Input: part model. Units: mm. Frame: model coordinates. Face numbers are marked on the shaded views. A direction names the side the tool comes from. Coordinates: 2 decimals unless noted, no trailing zeros. Loops run counter-clockwise (first coordinate to the right, second up) from the corner with the lowest first, then second, coordinate; pieces in that order, holes last.
Item 1: Pull-direction query (Z, two-part tool) for the marked faces 6, 7, 8 and 9; classes: released by +Z, released by -Z, zero draft, split by the parting line, or undercut.
Item 2: Ray query, line 1 along Z through (x, y) = (12.5, -0.25); line 2 along Z through (x, y) = (7, -4); line 3 along Y through (x, z) = (16, -21). Return the intervals inside material, ascending.
Item 3: Section D-D on x = 15. Return loops of the section in (y, z).
Item 4: Section A-A on z = -12.5. Return loops of the section in (x, y).
Item 5: Contact query for flat-ended pins moving along their axis: P1, Ø2, axis at x = 13.5, y = -2.5, coming from the +Z side; P2, Ø10, axis at x = 14, z = -12, coming from the -Y side; P3, Ø10, axis at x = 21, z = -16, coming from the -Y side; P4, Ø3, axis at x = 23.5, y = -2.5, coming from the -Z side. Output: stop coordinate, or through.
Item 6: Section C-C on x = 25. Return loops of the section in (y, z), and give its area (3 significant figures).
Item 7: Section B-B on y = -5.75. Return loops of the section in (x, z).
Item 8: Reachability of the marked faces 1, 2, 3, 4 and 5 from +Z, -Z, +X, -X, +Y, -Y: full face, straight path, thin tool, end or side. Return the list, or none.
```python
from build123d import *

# Parameters (mm, degrees)
BOSS_EXTRUDE1_DEPTH = 2
BOSS_EXTRUDE2_DEPTH = 2
SKETCH3_R           = 1
BOSS_EXTRUDE3_DEPTH = 2.5
SKETCH5_R           = 1
BOSS_EXTRUDE5_DEPTH = 2.5
SKETCH6_R           = 1
CUT_EXTRUDE1_DEPTH  = 2.5
BOSS_EXTRUDE6_START = -2.5
SKETCH8_R           = 1
BOSS_EXTRUDE6_DEPTH = 2.5
CUT_EXTRUDE2_DEPTH  = 2.5
SKETCH10_R          = 9.941576331
SKETCH10_R_2        = 9.5
BOSS_EXTRUDE9_DEPTH = 2.5


with BuildPart() as part:
    # Sketch1 → Boss-Extrude1 (new body)
    with BuildSketch(Plane(origin=(0, 0, 0), x_dir=(1, 0, 0), z_dir=(0, 1, 0))):
        Polygon((0, 2.5), (0, 0), (26, 0), (26, 25), (0, 25), (0, 22.5), (5, 22.5), (5, 2.5), align=None)
    extrude(amount=BOSS_EXTRUDE1_DEPTH)

    # Sketch2 → Boss-Extrude2 (add)
    with BuildSketch(Plane(origin=(0, 2, 0), x_dir=(1, 0, 0), z_dir=(0, 1, 0))):
        Polygon((26, 25), (40.579221248, 15.4966373), (40.579221248, 9.198619924), (26, 0), align=None)
    extrude(amount=-BOSS_EXTRUDE2_DEPTH)

    # Sketch3 → Boss-Extrude3 (add)
    with BuildSketch(Plane.XY):
        Polygon((15.962952465, 0), (0, 0), (0, -7.986136178), (3.187790207, -7.986136178), align=None)
        with Locations((1.984518411, -4.657937593)):
            Circle(SKETCH3_R, mode=Mode.SUBTRACT)
    extrude(amount=-BOSS_EXTRUDE3_DEPTH)

    # Sketch5 → Boss-Extrude5 (add)
    with BuildSketch(Plane.XY):
        with Locations((1.984518411, -4.657937593)):
            Circle(SKETCH5_R)
    extrude(amount=-BOSS_EXTRUDE5_DEPTH)

    # Sketch6 → Cut-Extrude1 (cut)
    with BuildSketch(Plane.XY):
        with Locations((1.984518411, -3.146677254)):
            Circle(SKETCH6_R)
    extrude(amount=-CUT_EXTRUDE1_DEPTH, mode=Mode.SUBTRACT)

    # Sketch8 → Boss-Extrude6 (add)
    with BuildSketch(Plane(origin=(0, 0, -25), x_dir=(-1, 0, 0), z_dir=(0, 0, -1)).offset(BOSS_EXTRUDE6_START)):
        Polygon((0, 0), (0, -7.986136178), (-3.187790207, -7.986136178), (-15.962952465, 0), align=None)
        with Locations(Location((-1.984518411, -3.146677254, 0), (0, 0, 180))):
            Circle(SKETCH8_R, mode=Mode.SUBTRACT)
    extrude(amount=BOSS_EXTRUDE6_DEPTH)

    # Sketch9 → Cut-Extrude2 (cut)
    with BuildSketch(Plane(origin=(0, 2, 0), x_dir=(1, 0, 0), z_dir=(0, 1, 0))):
        Polygon((21.748897696, 25), (29.198942219, 16.980267325), (29.198942219, 8.019732675), (21.748897696, 0), (26, 0), (40.579221248, 9.198619924), (40.579221248, 15.4966373), (26, 25), align=None)
    extrude(amount=-CUT_EXTRUDE2_DEPTH, mode=Mode.SUBTRACT)

    # Sketch10 → Boss-Extrude9 (add)
    with BuildSketch(Plane.XZ):
        with Locations(Location((18.089845789, -12.5, 0), (0, 0, 90))):
            Circle(SKETCH10_R)
        with Locations(Location((18.089845789, -12.5, 0), (0, 0, 270))):
            Circle(SKETCH10_R_2, mode=Mode.SUBTRACT)
    extrude(amount=BOSS_EXTRUDE9_DEPTH)


solid = part.part
```
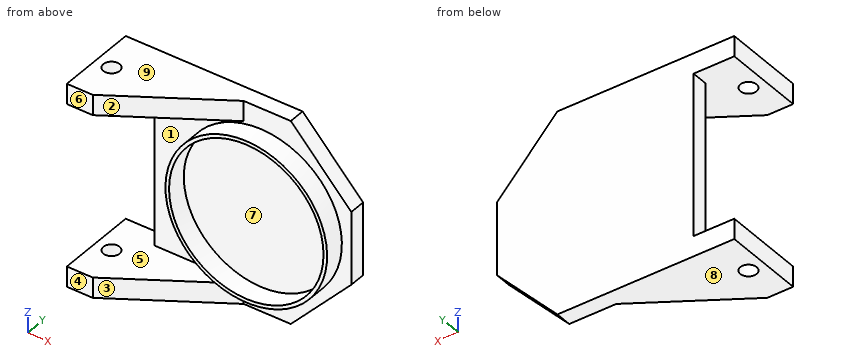
Results found:
1. face 6: zero draft
1. face 7: undercut
1. face 8: released by -Z
1. face 9: released by +Z
2. line 1: z = -25 to -22.5, -20.72 to -20.18, -4.82 to -4.28, -2.5 to 0
2. line 2: z = -25 to -22.5, -2.5 to 0
2. line 3: y = 0 to 2
3. outline: (-2.5, -21.95) - (0, -21.95) - (0, -22.5) - (-0.6, -22.5) - (-0.6, -25) - (2, -25) - (2, 0) - (-0.6, 0) - (-0.6, -2.5) - (0, -2.5) - (0, -3.05) - (-2.5, -3.05) - (-2.5, -3.52) - (0, -3.52) - (0, -21.48) - (-2.5, -21.48) - close
4. outline: (5, 0) - (8.15, 0) - (8.15, -2.5) - (8.59, -2.5) - (8.59, 0) - (27.59, 0) - (27.59, -2.5) - (28.03, -2.5) - (28.03, 0) - (29.2, 0) - (29.2, 2) - (5, 2) - close
5. P1: stops at z = 0
5. P2: stops at y = 0
5. P3: stops at y = -2.5
5. P4: stops at z = -21.64
6. outline: (-2.5, -19.65) - (0, -19.65) - (0, -21.5) - (2, -21.5) - (2, -3.5) - (0, -3.5) - (0, -5.35) - (-2.5, -5.35) - (-2.5, -5.98) - (0, -5.98) - (0, -19.02) - (-2.5, -19.02) - close
6. area: 39.1 mm2
7. outline: (0, -25) - (6.76, -25) - (6.76, -22.5) - (0, -22.5) - close; (0, -2.5) - (6.76, -2.5) - (6.76, 0) - (0, 0) - close
8. face 1: -Y
8. face 2: +Z, +X, -Y
8. face 3: -Z, +X, -Y
8. face 4: +Z, -Z, +X, -X, -Y
8. face 5: -X, -Y
